The model under review builds one solid part; all positions refer to its coordinate system, in mm. Face numbers are marked on the shaded views. A direction names the side the tool comes from. Coordinates: 2 decimals unless noted, no trailing zeros. Write each loop counter-clockwise with the first axis right and the second up, starting at its lowest first coordinate (ties: lowest second). Pieces come first, ordered by that corner, then holes.
Autodesk Inventor part; units mm, degrees
ref_plane "YZ Plane" through (0, 0, 0) normal (1, 0, 0) x (0, 1, 0)
ref_plane "XZ Plane" through (0, 0, 0) normal (0, 1, 0) x (-1, 0, 0)
ref_plane "XY Plane" through (0, 0, 0) normal (0, 0, 1) x (1, 0, 0)
sketch "스케치1" plane through (0, 0, 0) normal (0, 0, 1) x (1, 0, 0)
  line L0 (0, 0) -> (63.841, 0)
  line L1 (63.841, 0) -> (63.841, 6)
  line L2 (0, 6) -> (63.841, 6)
  line L3 (0, 0) -> (0, 6)
  line L4 (46.0408, 0) -> (46.0408, -150)
  line L5 (46.0408, -150) -> (51.8408, -150)
  line L6 (51.8408, -150) -> (51.8408, 0)
  line L7 (51.8408, 0) -> (46.0408, 0)
  line L8 (51.8408, 0) -> (63.841, 0)
  line L9 (63.841, 0) -> (63.841, -6)
  line L10 (63.841, -6) -> (51.8408, -6)
  line L11 (51.8408, -6) -> (51.8408, 0)
  line L12 (57.8409, 0) -> (51.8408, 0)
  line L13 (51.8408, 0) -> (51.8408, -12)
  line L14 (51.8408, -12) -> (57.8409, -12)
  line L15 (57.8409, -12) -> (57.8409, 0)
  point P0 (57.8409, -6)
extrude "돌출1" add sketch "스케치1" against normal blind 12 contours L0 L15 L10 L6 | L0 L9 L10 L15 | L10 L15 L14 L6
sketch "스케치2" plane through (0, 0, 0) normal (0, 0, 1) x (1, 0, 0)
  line L0 (63.841, -6) -> (57.8409, -6)
  line L1 (51.8408, 0) -> (63.841, 0)
  line L2 (57.8409, -6) -> (51.8408, -6)
  line L3 (51.8408, -6) -> (51.8408, 0)
  line L4 (51.8408, 0) -> (57.8409, 0)
  line L5 (57.8409, 0) -> (57.8409, -6)
  circle A0 centre (54.8408, -3) radius 1.45
  point P0 (0, 0)
extrude "돌출2" cut sketch "스케치2" against normal up to next contours A0
sketch "스케치3" plane through (57.8409, -6, 0) normal (0, -1, 0) x (1, 0, 0)
  line L0 (6.0001, 0) -> (-6.0001, 0)
  line L1 (0, 0) -> (0, -12)
  line L2 (6.0001, 0) -> (0, 0)
  line L3 (0, 0) -> (0, -6)
  line L4 (0, -6) -> (6.0001, -6)
  line L5 (6.0001, -6) -> (6.0001, 0)
  circle A0 centre (3.0001, -3) radius 1.35
  point P0 (-57.8409, 0)
  dimension "d6" = 2.7
extrude "돌출3" cut sketch "스케치3" against normal up to next contours A0
sketch "스케치4" plane through (57.8409, -12, 0) normal (1, 0, 0) x (0, 0, -1)
  line L0 (12, 6) -> (12, 0)
  line L1 (0, 6) -> (12, 6)
  line L2 (12, 0) -> (6, 0)
  line L3 (6, 0) -> (6, 6)
  line L4 (6, 6) -> (12, 6)
  line L5 (12, 6) -> (12, 0)
  circle A0 centre (9, 3) radius 1.35
  point P0 (0, 12)
  dimension "d9" = 2.7
extrude "돌출4" cut sketch "스케치4" against normal up to next contours A0
properties part number "부품75"
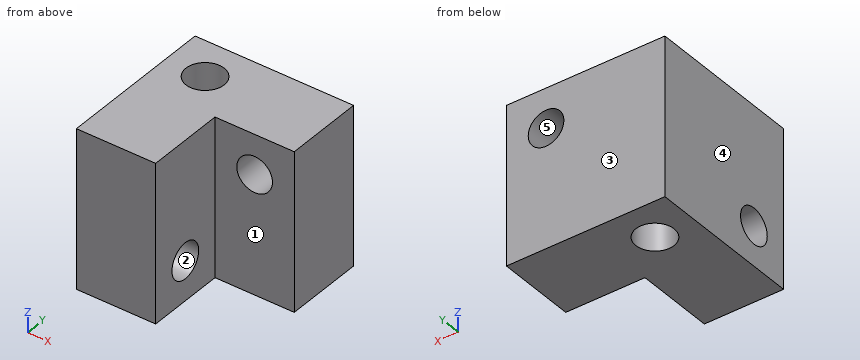
Item 1: Take a section at B-B, the plane z = -9. Write out the cut boundary in (x, y).
Solved:
outline: (51.84, -12) - (57.84, -12) - (57.84, -10.35) - (51.84, -10.35) - close; (51.84, -7.65) - (57.84, -7.65) - (57.84, -6) - (63.84, -6) - (63.84, 0) - (51.84, 0) - close; hole circle Ø2.9 at (54.84, -3)
Item 2: Mouldability with a two-part tool opening along X and no side actions: class the marked faces 3, 4 and 5 as pulls with the +X half, pulls with the -X half, needs draft (parallel to the pull), parting line crosses it, or undercut.
Solved:
face 3: needs draft
face 4: pulls with the -X half
face 5: undercut
Item 3: For pin 1 (6.5 mm diameter, centred on x = 61.5, z = -9, fed in from -Y), flat-tipped, find the tip position at first contact; note if it passes through.
Solved:
pin 1: stops at y = -6
Item 4: Take a section at C-C, the plane z = -11. Write out the cut boundary in (x, y), plus the area to 3 significant figures.
Solved:
outline: (51.84, -12) - (57.84, -12) - (57.84, -6) - (63.84, -6) - (63.84, 0) - (51.84, 0) - close; hole circle Ø2.9 at (54.84, -3)
area: 101 mm2
Item 5: Take a section at A-A, the plane y = -3. Write out the cut boundary in (x, z).
Solved:
outline: (51.84, -12) - (53.39, -12) - (53.39, 0) - (51.84, 0) - close; (56.29, -12) - (63.84, -12) - (63.84, 0) - (56.29, 0) - close; hole circle Ø2.7 at (60.84, -3)
Item 6: To check wall thickness, follow line 1 along Y through (x, z) = (55.25, -9); line 2 along Y through (x, z) = (56, -9); line 3 along Y through (x, z) = (59, -3.5). State the ranges of each line that lie inside material, in increasing order.
Solved:
line 1: y = -12 to -10.35, -7.65 to -4.39, -1.61 to 0
line 2: y = -12 to -10.35, -7.65 to -3.87, -2.13 to 0
line 3: y = -6 to 0
Item 7: Take a section at D-D, the plane y = -9. Write out the cut boundary in (x, z).
Solved:
outline: (51.84, -12) - (57.84, -12) - (57.84, -10.35) - (51.84, -10.35) - close; (51.84, -7.65) - (57.84, -7.65) - (57.84, 0) - (51.84, 0) - close
Item 8: Machinability: for the marked faces 1 and 2, which of the approach directions +Z, -Z, +X, -X, +Y, -Y give a long, thin tool a straight path to every point of the face, cutting with its end or side? Answer none if there is none.
Solved:
face 1: +Z, -Z, +X, -Y
face 2: +X, -X
